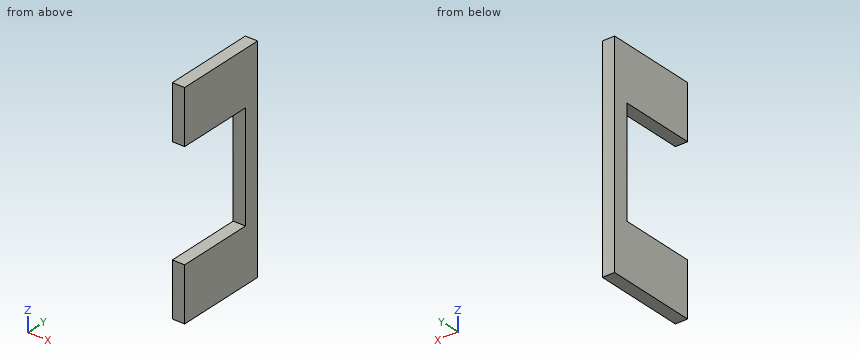
Autodesk Inventor part; units mm, degrees
ref_plane "YZ Plane" through (0, 0, 0) normal (1, 0, 0) x (0, 1, 0)
ref_plane "XZ Plane" through (0, 0, 0) normal (0, 1, 0) x (-1, 0, 0)
ref_plane "XY Plane" through (0, 0, 0) normal (0, 0, 1) x (1, 0, 0)
sketch "Эскиз1" plane through (0, 0, 0) normal (0, 1, 0) x (-1, 0, 0)
  line L0 (0, 0) -> (4, 0)
  line L1 (4, 0) -> (4, 70)
  line L2 (4, 70) -> (0, 70)
  line L3 (0, 70) -> (0, 0)
  dimension "d0" = 4
  dimension "d1" = 70
extrude "Выдавливание1" add sketch "Эскиз1" along normal blind 30
sketch "Эскиз2" plane through (0, 0, 70) normal (1, 0, 0) x (0, 0, -1)
  line L0 (70, 0) -> (0, 0)
  line L1 (17.5, 0) -> (52.5, 0)
  line L2 (52.5, 0) -> (52.5, 25)
  line L3 (52.5, 25) -> (17.5, 25)
  line L4 (17.5, 25) -> (17.5, 0)
  point P0 (35, 0)
  dimension "d4" = 35
  dimension "d5" = 25
extrude "Выдавливание2" cut sketch "Эскиз2" against normal blind 30
properties part number "перед"
For this review, take the finished solid that the model builds, in its own axes (mm). Give positions to 0.01 mm unless a question says otherwise; leave off trailing zeros. Order: outer loops, then holes, each group sorted by start corner. A loop starts at its lowest first (then second) coordinate and runs counter-clockwise, first axis right, second up. Notation, with made-up numbers: (70.5, 7.25) - (84.5, 7.25) arc R26 cw to (84.5, 21.25) - close; hole circle Ø1 at (-14, 36.5). An arc over 180 degrees is marked (long way). Answer as a JSON object with one key per item and string values. Group by question number.
Item 1: Take a section at A-A on x = -2.25. Give the boundary of the cut face in (y, z), and give its area (4 significant figures).
Item 2: Clearance check with a flat-ended pin moving along its axis: pin 1 Ø1.2 at (x, z) = (-1.5, 34.5) entering from -Y. State where the tip first meets the part, or that it passes through.
Item 3: Take a section at B-B on y = 19. Give the boundary of the cut face in (x, z).
Item 4: Take a section at C-C on z = 25. Give the boundary of the cut face in (x, y).
Item 5: Wall thickness on line 1 along Z through (x, y) = (-3.45, 2.75); line 2 along Y through (x, z) = (-0.15, 34.5): over which ranges is each line inside the solid? List them lowest first.
Reported:
{
 "1": {"outline": "(0, 0) - (30, 0) - (30, 70) - (0, 70) - (0, 52.5) - (25, 52.5) - (25, 17.5) - (0, 17.5) - close", "area": "1,225 mm^2"},
 "2": {"pin 1": "y = 25"},
 "3": {"outline": "(-4, 0) - (0, 0) - (0, 17.5) - (-4, 17.5) - close; (-4, 52.5) - (0, 52.5) - (0, 70) - (-4, 70) - close"},
 "4": {"outline": "(-4, 25) - (0, 25) - (0, 30) - (-4, 30) - close"},
 "5": {"line 1": "0 to 17.5, 52.5 to 70", "line 2": "25 to 30"}
}
